The model under review builds one solid part; all positions refer to its coordinate system, in mm. A direction names the side the tool comes from. Give positions to 0.01 mm unless a question says otherwise; leave off trailing zeros. Write each loop counter-clockwise with the first axis right and the second up, starting at its lowest first coordinate (ties: lowest second). Pieces come first, ordered by that corner, then holes. Notation, with made-up numbers: (58.25, 37.5) - (74.25, 37.5) arc R34 cw to (74.25, 74.5) - close; hole circle Ø5 at (72.25, 48). An arc over 180 degrees is marked (long way). Write item = value, one per line.
Autodesk Inventor part; units mm, degrees
ref_plane "YZ Plane" through (0, 0, 0) normal (1, 0, 0) x (0, 1, 0)
ref_plane "XZ Plane" through (0, 0, 0) normal (0, 1, 0) x (-1, 0, 0)
ref_plane "XY Plane" through (0, 0, 0) normal (0, 0, 1) x (1, 0, 0)
sketch "Sketch1" plane through (0, 0, 0) normal (0, 0, 1) x (1, 0, 0)
  circle A0 centre (0, 0) radius 19
  dimension "d0" = 38
extrude "Extrusion1" add sketch "Sketch1" along normal blind 6
sketch "Sketch2" plane through (0, 0, 6) normal (0, 0, 1) x (1, 0, 0)
  circle A0 centre (0, 0) radius 26
  dimension "d3" = 52
extrude "Extrusion2" add sketch "Sketch2" along normal blind 2.3
sketch "Sketch3" plane through (0, 0, 8.3) normal (0, 0, 1) x (1, 0, 0)
  circle A0 centre (0, 0) radius 16.5
  dimension "d6" = 33
extrude "Extrusion3" add sketch "Sketch3" along normal blind 0.5
sketch "Sketch4" plane through (0, 0, 8.8) normal (0, 0, 1) x (1, 0, 0)
  circle A0 centre (0, 0) radius 12.5
  dimension "d9" = 25
extrude "Extrusion4" add sketch "Sketch4" along normal blind 7.75
sketch "Sketch5" plane through (0, 0, 16.55) normal (0, 0, 1) x (1, 0, 0)
  circle A0 centre (0, 0) radius 8.25
  dimension "d12" = 16.5
extrude "Extrusion5" add sketch "Sketch5" along normal blind 2.5
sketch "Sketch6" plane through (0, 0, 16.55) normal (0, 0, 1) x (1, 0, 0)
  line L0 (0, -36.4) -> (0, 36.4)
  point P0 (0, 0)
  point P1 (0, 10.55)
  point P2 (-10.55, 0)
  point P3 (0, -10.55)
  point P4 (10.55, 0)
  dimension "d15" = 10.55
  dimension "d18" = 360
hole "Hole1" at (0, 10.55, 16.55) at (-10.55, 0, 16.55) at (0, -10.55, 16.55) at (10.55, 0, 16.55) direction (0, 0, -1) diameter 1.7129 depth 5
sketch "Sketch7" plane through (0, 0, 19.05) normal (0, 0, 1) x (1, 0, 0)
  circle A0 centre (0, 0) radius 1.5
  dimension "d27" = 3
extrude "Extrusion6" cut sketch "Sketch7" against normal through all
properties part number "motor"
1. For line 1 (Y direction, x = 0, z = 12.25); line 2 (Y direction, x = 0, z = 10); line 3 (Z direction, x = 23.5, y = 0.5), list the stretches that pass through material, from the lowest coordinate up. Write a range as from..to.
Findings below:
line_1 = -12.5..-11.41, -9.69..-1.5, 1.5..9.69, 11.41..12.5
line_2 = -12.5..-1.5, 1.5..12.5
line_3 = 6..8.3
2. Take a section at C-C on z = 10. Give the boundary of the cut face in (x, y), and give its area (3 significant figures).
Findings below:
outline = circle Ø25 at (0, 0); hole circle Ø3 at (0, 0)
area = 484 mm²
3. Take a section at D-D on y = -10.55. Give the boundary of the cut face in (x, z), and give its area (3 significant figures).
Findings below:
outline = (-23.76, 6) - (-15.8, 6) - (-15.8, 0) - (15.8, 0) - (15.8, 6) - (23.76, 6) - (23.76, 8.3) - (12.69, 8.3) - (12.69, 8.8) - (6.7, 8.8) - (6.7, 16.55) - (0.86, 16.55) - (0.86, 11.55) - (-0.86, 11.55) - (-0.86, 16.55) - (-6.7, 16.55) - (-6.7, 8.8) - (-12.69, 8.8) - (-12.69, 8.3) - (-23.76, 8.3) - close
area = 407 mm²
4. Machinability: for faces 1 (the cylindrical face through (-20.633, 15.821, 7.134)), 2 (the cylindrical face through (7.62, 3.16, 17.78)), 3 (the flat face through (1.8, -19.1, 6)), which of the approach directions +Z, -Z, +X, -X, +Y, -Y give a long, thin tool a straight path to every point of the face, cutting with its end or side? Answer none if there is none.
Findings below:
face_1 = +Z, -Z
face_2 = +Z
face_3 = -Z
5. Insertion check: P1, Ø2, axis at x = -10.5, z = 11, coming from the -Y side; P2, Ø3, axis at y = 10, z = 2, coming from the -X side; P3, Ø8, axis at x = -2, y = -14, coming from the +Z side; P4, Ø2, axis at x = -3, y = 14, coming from the -Z side. Each pin has a flat end and moves straight along its axis. Give the tip position at first contact, or say it passes through.
Findings below:
P1 = -8.12
P2 = -16.99
P3 = 16.55
P4 = 0
6. Take a section at B-B on z = 13.5. Give the boundary of the cut face in (x, y).
Findings below:
outline = circle Ø25 at (0, 0); hole circle Ø1.71 at (-10.55, 0); hole circle Ø3 at (0, 0); hole circle Ø1.71 at (0, -10.55); hole circle Ø1.71 at (0, 10.55); hole circle Ø1.71 at (10.55, 0)
7. Draft analysis for pull direction Y (two halves, no side actions). For faces 4 (the cylindrical face through (8.767, 16.856, 2.958)), 5 (the cylindrical face through (0.33, -11.34, 14.02)), 6 (the flat face through (3, -8, 16.55)), state which applies: +Y half, -Y half, draft (parallel to the pull), parting line (faces both ways), or undercut.
Findings below:
face_4 = parting line
face_5 = undercut
face_6 = draft
